Here's how the part is built. I have some questions about the finished solid (model axes, mm). Round coordinates to 2 decimals unless told otherwise and drop trailing zeros. Loops run counter-clockwise (first coordinate to the right, second up) from the corner with the lowest first, then second, coordinate; pieces in that order, holes last. Notation, with made-up numbers: (84.25, -2) -> (91.25, -2) arc R23 cw to (91.25, 14) -> close; hole circle Ø7 at (47, 53.25). An arc over 180 degrees is marked (long way). One line per item, written item: value. Start each with the question number.
```python
from build123d import *

# Parameters (mm, degrees)
SKETCH_R    = 50
SKETCH_R_2  = 25
PAD_DEPTH   = 50
FILLET_R    = 20
FILLET001_R = 20


with BuildPart() as part:
    # Sketch → Pad (new body)
    with BuildSketch(Plane.XZ):
        Circle(SKETCH_R)
        Circle(SKETCH_R_2, mode=Mode.SUBTRACT)
    extrude(amount=PAD_DEPTH)

    # Fillet
    fillet_edges = [part.edges().sort_by_distance(p)[0] for p in [
        (-50, -50, 0),
    ]]
    fillet(fillet_edges, radius=FILLET_R)

    # Fillet001
    fillet001_edges = [part.edges().sort_by_distance(p)[0] for p in [
        (-50, 0, 0),
    ]]
    fillet(fillet001_edges, radius=FILLET001_R)


solid = part.part
```
Q1. Will these pins go through, and if not, where does the flat tip stop? P1, Ø6, axis at x = -18.5, y = -16.5, coming from the +Z side; P2, Ø6, axis at x = -33, y = -27.5, coming from the -Z side; P3, Ø4, axis at y = -14, z = 20.5, coming from the -X side.
Q2. I want a section at C-C on y = -8. Please give me the cut outline in (x, z).
Q3. If I drill on line 1 along Z through (x, y) = (0, -30); line 2 along Z through (x, y) = (0, -41); line 3 along X through (y, z) = (-18, 36.5), over which ranges is the centre line in solid material (lowest first)?
Q4. I want a section at B-B on x = 0. Please give me the cut outline in (y, z).
Q5. I want a section at D-D on y = -16.5. Please give me the cut outline in (x, z), plus the area to 3 significant figures.
Q6. If we mould it in two halves opening along X, with no side actions, what happens to faces 1 (the cylindrical face through (47.69, -24.93, 15.02)), 2 (the flat face through (-7, 0, 25)), 3 (the cylindrical face through (23.846, -24.65, 7.509))? For each: released by +X, released by -X, zero draft, split by the parting line, or undercut.
Q7. I want a section at A-A on z = 0. Please give me the cut outline in (x, y), plus the area to 3 significant figures.
Answers below:
1. P1: stops at z = 47.32
1. P2: stops at z = -40
1. P3: stops at x = -45.66
2. outline: circle Ø92 at (0, 0); hole circle Ø50 at (0, 0)
3. line 1: z = -50 to -25, 25 to 50
3. line 2: z = -46.7 to -25, 25 to 46.7
3. line 3: x = -34.03 to 34.03
4. outline: (-50, -30) arc R20 ccw to (-30, -50) -> (-20, -50) arc R20 ccw to (0, -30) -> (0, -25) -> (-50, -25) -> close; (-50, 25) -> (0, 25) -> (0, 30) arc R20 ccw to (-20, 50) -> (-30, 50) arc R20 ccw to (-50, 30) -> close
5. outline: circle Ø99.38 at (0, 0); hole circle Ø50 at (0, 0)
5. area: 5,790 mm^2
6. face 1: split by the parting line
6. face 2: zero draft
6. face 3: undercut
7. outline: (-50, -30) arc R20 ccw to (-30, -50) -> (-25, -50) -> (-25, 0) -> (-30, 0) arc R20 ccw to (-50, -20) -> close; (25, -50) -> (30, -50) arc R20 ccw to (50, -30) -> (50, -20) arc R20 ccw to (30, 0) -> (25, 0) -> close
7. area: 2,160 mm^2
